Design review of the part built by this model. Coordinates are the model's own, in mm. A direction names the side the tool comes from. Give positions to 0.01 mm unless a question says otherwise; leave off trailing zeros. Write each loop counter-clockwise with the first axis right and the second up, starting at its lowest first coordinate (ties: lowest second). Pieces come first, ordered by that corner, then holes. Notation, with made-up numbers: (88, -13.5) -> (110, -13.5) arc R20 cw to (110, 17.5) -> close; hole circle Ø2 at (19, -20). An arc over 180 degrees is marked (long way). Write each question's results on one line, items separated by ' | '. Start each with the question number.
(1) Mouldability with a two-part tool opening along Z and no side actions: class faces 1 (the face through (-8.43, -4.72, 0.27)), 2 (the face through (-6.4, -3.2, -1.4)), 3 (the face through (0.1, -11.2, 13)) as released by +Z, released by -Z, zero draft, split by the parting line, or undercut.
(2) To check wall thickness, follow probe 1 along Y at (x, z) = (7.7, 0); probe 2 along X at (y, z) = (-2.25, 1); probe 3 along Y at (x, z) = (-10, 5.25). State the ranges of each line that lie inside material, in increasing order.
(3) Take a section at B-B (z = -8.25). State the section outline as (x, y) points, plus the area to 3 significant figures.
(4) Clearance check with flat-ended pins moving along their axes: pin 1 (6 mm diameter, centred on x = 4, y = -9, fed in from -Z); pin 2 (1.8 mm diameter, centred on y = -2.5, z = 1.5, fed in from +X); pin 3 (3 mm diameter, centred on x = -0.5, z = -6.5, fed in from -Y). State where each tip first meets the part, or that it passes through.
(5) Take a section at A-A (z = 0). State the section outline as (x, y) points.
(6) Take a section at C-C (x = 1.75). State the section outline as (y, z) points.
(7) Take a section at D-D (y = -3). State the section outline as (x, z) points, plus the area to 3 significant figures.
(8) For faces 4 (the face through (-4.158, 0.507, -7.061)), 5 (the face through (-8, -3, -3)), 6 (the face through (0, -6, 12)), 7 (the face through (10.4, -3.2, -1.4)), list the 3-axis set-ups (+Z, -Z, +X, -X, +Y, -Y) from which the entire face can be reached by the end or side of a thin tool; tool diameter is ignored.
from build123d import *

# Parameters (mm, degrees)
SKIZZE1_W                       = 23
SKIZZE1_H                       = 26
AUFSATZ_LINEAR_AUSTRAGEN1_DEPTH = 1
SKIZZE2_W                       = 4
SKIZZE2_H                       = 6
AUFSATZ_LINEAR_AUSTRAGEN2_DEPTH = 6.5
SKIZZE3_R                       = 1.25
SCHNITT_LINEAR_AUSTRAGEN1_DEPTH = 4
AUFSATZ_LINEAR_AUSTRAGEN3_DEPTH = 1
AUFSATZ_LINEAR_AUSTRAGEN4_DEPTH = 1
SCHNITT_LINEAR_AUSTRAGEN2_DEPTH = 1
VERRUNDUNG1_R                   = 1


with BuildPart() as part:
    # Skizze1 → Aufsatz-Linear austragen1 (new body)
    with BuildSketch(Plane(origin=(0, 0, 0), x_dir=(1, 0, 0), z_dir=(0, 1, 0))):
        Rectangle(SKIZZE1_W, SKIZZE1_H)
    extrude(amount=AUFSATZ_LINEAR_AUSTRAGEN1_DEPTH)

    # Skizze2 → Aufsatz-Linear austragen2 (add)
    with BuildSketch(Plane.XZ):
        with Locations((8.4, 0)):
            Rectangle(SKIZZE2_W, SKIZZE2_H)
    aufsatz_linear_austragen2 = extrude(amount=AUFSATZ_LINEAR_AUSTRAGEN2_DEPTH)

    # Skizze3 → Schnitt-Linear austragen1 (cut)
    with BuildSketch(Plane(origin=(10.4, 0, 0), x_dir=(0, 0, -1), z_dir=(1, 0, 0))):
        with Locations((0, -3.5)):
            Circle(SKIZZE3_R)
    schnitt_linear_austragen1 = extrude(amount=-SCHNITT_LINEAR_AUSTRAGEN1_DEPTH, mode=Mode.SUBTRACT)

    # Spiegeln1: Aufsatz-Linear austragen2, Schnitt-Linear austragen1 across plane
    add(aufsatz_linear_austragen2.mirror(Plane(origin=(0, 0, 0), x_dir=(0, 0, 1), z_dir=(1, 0, 0))))
    add(schnitt_linear_austragen1.mirror(Plane(origin=(0, 0, 0), x_dir=(0, 0, 1), z_dir=(1, 0, 0))), mode=Mode.SUBTRACT)

    # Skizze4 → Aufsatz-Linear austragen3 (add)
    with BuildSketch(Plane.XY.offset(13)):
        Polygon((9.9, 1), (-9.9, 1), (-7.9, -10.9), (7.9, -10.9), align=None)
    extrude(amount=AUFSATZ_LINEAR_AUSTRAGEN3_DEPTH)

    # Skizze5 → Aufsatz-Linear austragen4 (add)
    with BuildSketch(Plane(origin=(0, 0, 13), x_dir=(-1, 0, 0), z_dir=(0, 0, -1))):
        Polygon((-7.9, -11.9), (7.9, -11.9), (9.9, 0), (-9.9, 0), align=None)
    extrude(amount=AUFSATZ_LINEAR_AUSTRAGEN4_DEPTH)

    # Skizze6 → Schnitt-Linear austragen2 (cut)
    with BuildSketch(Plane(origin=(0, 1, 0), x_dir=(1, 0, 0), z_dir=(0, 1, 0))):
        with BuildLine():
            Line((3.3, 9.9), (-3.3, 9.9))
            ThreePointArc((-3.3, 9.9), (-4.148528137, 9.548528137), (-4.5, 8.7))
            Line((-4.5, 8.7), (-4.5, 7.9))
            ThreePointArc((-4.5, 7.9), (-4.148528137, 7.051471863), (-3.3, 6.7))
            Line((-3.3, 6.7), (3.3, 6.7))
            ThreePointArc((3.3, 6.7), (4.148528137, 7.051471863), (4.5, 7.9))
            Line((4.5, 7.9), (4.5, 8.7))
            ThreePointArc((4.5, 8.7), (4.148528137, 9.548528137), (3.3, 9.9))
        make_face()
    extrude(amount=-SCHNITT_LINEAR_AUSTRAGEN2_DEPTH, mode=Mode.SUBTRACT)

    # Verrundung1
    verrundung1_edges = [part.edges().sort_by_distance(p)[0] for p in [
        (0, 1, 14),
    ]]
    fillet(verrundung1_edges, radius=VERRUNDUNG1_R)


solid = part.part
Report:
1) face 1: undercut | face 2: zero draft | face 3: released by +Z
2) probe 1: -6.5 to -4.75, -2.25 to 1 | probe 2: -10.4 to -6.4, 6.4 to 10.4 | probe 3: 0 to 1
3) outline: (-11.5, 0) -> (-4.5, 0) -> (-4.5, 1) -> (-11.5, 1) -> close; (4.5, 0) -> (11.5, 0) -> (11.5, 1) -> (4.5, 1) -> close | area: 14.0 mm2
4) pin 1: z = 12 | pin 2: x = 10.4 | pin 3: y = 0
5) outline: (-11.5, 0) -> (-10.4, 0) -> (-10.4, -2.25) -> (-6.4, -2.25) -> (-6.4, 0) -> (6.4, 0) -> (6.4, -2.25) -> (10.4, -2.25) -> (10.4, 0) -> (11.5, 0) -> (11.5, 1) -> (-11.5, 1) -> close; (-10.4, -6.5) -> (-6.4, -6.5) -> (-6.4, -4.75) -> (-10.4, -4.75) -> close; (6.4, -6.5) -> (10.4, -6.5) -> (10.4, -4.75) -> (6.4, -4.75) -> close
6) outline: (-11.9, 12) -> (0, 12) -> (0, -6.7) -> (1, -6.7) -> (1, 13) arc R1 ccw to (0, 14) -> (-10.9, 14) -> (-10.9, 13) -> (-11.9, 13) -> close; (0, -13) -> (1, -13) -> (1, -9.9) -> (0, -9.9) -> close
7) outline: (-10.4, -3) -> (-6.4, -3) -> (-6.4, -1.15) -> (-10.4, -1.15) -> close; (-10.4, 1.15) -> (-6.4, 1.15) -> (-6.4, 3) -> (-10.4, 3) -> close; (-9.4, 12) -> (9.4, 12) -> (9.4, 13) -> (9.23, 13) -> (9.23, 14) -> (-9.23, 14) -> (-9.23, 13) -> (-9.4, 13) -> close; (6.4, -3) -> (10.4, -3) -> (10.4, -1.15) -> (6.4, -1.15) -> close; (6.4, 1.15) -> (10.4, 1.15) -> (10.4, 3) -> (6.4, 3) -> close | area: 66.9 mm2
8) face 4: +Y, -Y | face 5: -Z, +X, -X, -Y | face 6: +X, -X, -Y | face 7: +Z, -Z, +X, -Y
